Work out the finished part from the listing and answer in its coordinate system (mm). A direction names the side the tool comes from. Give positions to 0.01 mm unless a question says otherwise; leave off trailing zeros. Order: outer loops, then holes, each group sorted by start corner. A loop starts at its lowest first (then second) coordinate and runs counter-clockwise, first axis right, second up. Notation, with made-up numbers: (21, 24.25) - (60, 24.25) arc R21 cw to (60, 50.25) - close; hole circle Ø8 at (-16.5, 63). An arc over 180 degrees is marked (long way). Write each question's results on one line, items separated by ' | '.
from build123d import *

# Parameters (mm, degrees)
F0_R     = 15.5
F1_DEPTH = 8
F2_T     = -5
F3_R     = 1.5
F4_R     = 1.2


with BuildPart() as f1:
    # F0 (on Top) → F1 (new body)
    with BuildSketch(Plane.XY):
        with Locations((-16.122315079, 8.5424212739)):
            Circle(F0_R)
    extrude(amount=F1_DEPTH)

    # F2
    f2_openings = [f1.faces().sort_by_distance(p)[0] for p in [
        (-16.122315, 8.542421, 0),
    ]]
    offset(amount=F2_T, openings=f2_openings)

    # F3
    f3_edges = [f1.edges().sort_by_distance(p)[0] for p in [
        (-31.622315, 8.542421, 0),
    ]]
    fillet(f3_edges, radius=F3_R)

    # F4
    f4_edges = [f1.edges().sort_by_distance(p)[0] for p in [
        (-26.622315, 8.542421, 0),
        (-1.061655, 8.542421, 0.43934),
        (-31.622315, 8.542421, 1.5),
        (-30.122315, 8.542421, 0),
    ]]
    fillet(f4_edges, radius=F4_R)


solid = f1.part
1. A tool of negligible diameter and unlimited length cuts with its end or side. For faces 4 (the face through (-16, 9, 3)), 5 (the face through (-19, -3, 0)), from which of +Z, -Z, +X, -X, +Y, -Y can it reach the whole face along a straight path? Write none if from no direction.
Answer list:
face 4: -Z | face 5: -Z, +X, -X, +Y, -Y
2. Given P1, Ø1.5, axis at x = -8, y = 10, coming from the -Z side; P2, Ø1.5, axis at x = -8.5, z = 4, coming from the +Y side, each flat-ended and moving along its own axis, determine where each tip first touches the part or whether it passes through.
Answer list:
P1: z = 3 | P2: y = 22.44
3. A cutting plane is placed at A-A, the plane z = 2.5. Write down the section's boundary in (x, y), then the cut area to 3 significant figures.
Answer list:
outline: circle Ø31 at (-16.12, 8.54); hole circle Ø21 at (-16.12, 8.54) | area: 408 mm^2
4. A cutting plane is placed at B-B, the plane z = 7.5. Write down the section's boundary in (x, y).
Answer list:
outline: circle Ø31 at (-16.12, 8.54)
5. Determine the mould class of faces 1 (the face through (-16, 9, 8)), 2 (the face through (-1.804, 2.606, 4.704)), 3 (the face through (-11.277, -0.773, 2.087)) for opening direction Y: +Y half, -Y half, draft (parallel to the pull), parting line (faces both ways), or undercut.
Answer list:
face 1: draft | face 2: parting line | face 3: undercut
6. Straight lines are drawn through the part: line 1 (X direction, y = 16.5, z = 2); line 2 (Z direction, x = -13, y = 10); line 3 (Y direction, x = -22, z = 1.75). For each, find the intervals that lie inside material, in ascending order. Write a range as [from, to].
Answer list:
line 1: [-29.42, -22.97], [-9.27, -2.82] | line 2: [3, 8] | line 3: [-5.8, -0.16], [17.24, 22.88]
